Can you work these out from the model? Positions are in its coordinate system, mm. A direction names the side the tool comes from. Coordinates: 2 decimals unless noted, no trailing zeros. Write each loop counter-clockwise with the first axis right and the second up, starting at its lowest first coordinate (ties: lowest second). Pieces come first, ordered by that corner, then holes. Notation, with made-up numbers: (-20.75, 39.5) - (35.25, 39.5) arc R26 ccw to (35.25, 56.5) - close; hole circle Ø7 at (77, -14). An arc over 180 degrees is marked (long way). Use one line per item in the form item = value. Start each with the question number.
(1) If we section it at B-B on z = 4.25: Please give me the cut outline in (x, y), then the cut area to 3 significant figures.
(2) On a 3-axis mill with a long thin cutter (end or side, diameter ignored), from which of +Z, -Z, +X, -X, +Y, -Y can I reach the whole of each face in a straight line? I mean faces 1 (the face through (37.3, 22, 4.9)), 2 (the face through (37.675, -21.348, 4.93)), 3 (the face through (51, 15, 15)), 4 (the face through (49, 0, 25)). Say none if no direction works.
(3) If I drill on probe 1 along X at (y, z) = (-2, 17.25); probe 2 along Z at (x, y) = (30, 20); probe 3 along Z at (x, y) = (20, 12), over which ranges is the centre line in solid material (lowest first)? Write a range as from..to.
(4) For pin 1 Ø11 at (x, z) = (34, 17) entering from +Y; pin 2 Ø5 at (x, z) = (52.5, 15.5) entering from -Y; pin 3 Ø6 at (x, y) = (1.5, -9) entering from +Z, each with a flat end and sliding along its axis, tell me the tip position at first contact or that it passes through.
(5) If we section it at C-C on y = 18: Please give me the cut outline in (x, z), then the cut area to 3 significant figures.
(6) If we section it at A-A on x = 55: Please give me the cut outline in (y, z).
(7) If we section it at D-D on x = 34: Please give me the cut outline in (y, z), then the cut area to 3 significant figures.
Autodesk Inventor part; units mm, degrees
ref_plane "YZ Plane" through (0, 0, 0) normal (1, 0, 0) x (0, 1, 0)
ref_plane "XZ Plane" through (0, 0, 0) normal (0, 1, 0) x (-1, 0, 0)
ref_plane "XY Plane" through (0, 0, 0) normal (0, 0, 1) x (1, 0, 0)
sketch "Boceto1" plane through (0, 0, 0) normal (0, 0, 1) x (1, 0, 0)
  line L0 (50, 0) -> (25, -43.3013)
  line L1 (25, -43.3013) -> (-25, -43.3013)
  line L2 (-25, -43.3013) -> (-50, 0)
  line L3 (-50, 0) -> (-25, 43.3013)
  line L4 (-25, 43.3013) -> (25, 43.3013)
  line L5 (25, 43.3013) -> (50, 0)
  point P0 (0, 0)
  point P1 (0, 0)
  dimension "d3" = 50
extrude "Extrusión1" add sketch "Boceto1" along normal blind 10
sketch "Boceto2" plane through (0, 0, 10) normal (0, 0, 1) x (1, 0, 0)
  line L0 (13.773, -15) -> (86.227, -15)
  line L1 (86.227, -15) -> (86.227, 15)
  line L2 (86.227, 15) -> (13.773, 15)
  line L3 (13.773, 15) -> (13.773, -15)
  line L4 (25, -43.3013) -> (50, 0)
  line L5 (13.773, -15) -> (86.227, 15) construction
  line L6 (86.227, -15) -> (13.773, 15) construction
  dimension "d7" = 30
  dimension "d8" = 72.454
extrude "Extrusión2" add sketch "Boceto2" along normal blind 10
sketch "Boceto3" plane through (0, 0, 20) normal (0, 0, 1) x (1, 0, 0)
  line L0 (13.773, 15) -> (41.3397, 15)
  line L1 (41.3397, 15) -> (25, 43.3013)
  line L2 (25, 43.3013) -> (-25, 43.3013)
  line L3 (-25, 43.3013) -> (-50, 0)
  line L4 (-50, 0) -> (-25, -43.3013)
  line L5 (-25, -43.3013) -> (25, -43.3013)
  line L6 (25, -43.3013) -> (41.3397, -15)
  line L7 (41.3397, -15) -> (13.773, -15)
  line L8 (13.773, -15) -> (13.773, 15)
  line L9 (0, 0) -> (55, 0)
  circle A0 centre (55, 0) radius 6
  line L10 (13.773, 15) -> (41.3397, 15)
  line L11 (41.3397, 15) -> (25, 43.3013)
  line L12 (25, 43.3013) -> (-25, 43.3013)
  line L13 (-25, 43.3013) -> (-50, 0)
  line L14 (-50, 0) -> (-25, -43.3013)
  line L15 (-25, -43.3013) -> (25, -43.3013)
  line L16 (25, -43.3013) -> (41.3397, -15)
  line L17 (41.3397, -15) -> (13.773, -15)
  line L18 (13.773, -15) -> (13.773, 15)
  line L19 (13.773, 15) -> (41.3397, 15)
  line L20 (41.3397, 15) -> (25, 43.3013)
  line L21 (25, 43.3013) -> (-25, 43.3013)
  line L22 (-25, 43.3013) -> (-50, 0)
  line L23 (-50, 0) -> (-25, -43.3013)
  line L24 (-25, -43.3013) -> (25, -43.3013)
  line L25 (25, -43.3013) -> (41.3397, -15)
  line L26 (41.3397, -15) -> (13.773, -15)
  line L27 (13.773, -15) -> (13.773, 15)
  line L28 (86.227, 15) -> (13.773, 15)
  dimension "d9" = 55
  dimension "d10" = 12
extrude "Extrusión3" add sketch "Boceto3" along normal blind 10 contours A0
properties part number "base"
Reported:
q1.outline = (-50, 0) - (-25, -43.3) - (25, -43.3) - (50, 0) - (25, 43.3) - (-25, 43.3) - close
q1.area = 6,500 mm2
q2.face_1 = -Z, +X, +Y
q2.face_2 = -Z, +X, -Y
q2.face_3 = +Z, +X, -X, +Y
q2.face_4 = +Z
q3.probe_1 = 13.77..86.23
q3.probe_2 = 0..10
q3.probe_3 = 0..20
q4.pin_1 = 15
q4.pin_2 = -15
q4.pin_3 = 10
q5.outline = (-39.61, 0) - (39.61, 0) - (39.61, 10) - (-39.61, 10) - close
q5.area = 792 mm2
q6.outline = (-15, 10) - (15, 10) - (15, 20) - (6, 20) - (6, 30) - (-6, 30) - (-6, 20) - (-15, 20) - close
q7.outline = (-27.71, 0) - (27.71, 0) - (27.71, 10) - (15, 10) - (15, 20) - (-15, 20) - (-15, 10) - (-27.71, 10) - close
q7.area = 854 mm2
